For this review, take the finished solid that the model builds, in its own axes (mm). A direction names the side the tool comes from. Give positions to 0.01 mm unless a question says otherwise; leave off trailing zeros. Loops run counter-clockwise (first coordinate to the right, second up) from the corner with the lowest first, then second, coordinate; pieces in that order, holes last. Notation, with made-up numbers: (30.5, 54) - (58.5, 54) arc R28 cw to (58.5, 91) - close; hole circle Ø3 at (-21.5, 73.5). An arc over 180 degrees is marked (long way). Put each result on its own line as item: value.
from build123d import *

# Parameters (mm, degrees)
F0_W     = 935.182943
F0_H     = 745.169759
F1_DEPTH = 25
F2_W     = 160
F2_H     = 100
F3_DEPTH = 131.70007
F5_D     = 20
F6_R     = 71.842191


with BuildPart() as f1:
    # F0 (on Top) → F1 (new body)
    with BuildSketch(Plane.XY):
        with Locations((-262.850217, -86.583943)):
            Rectangle(F0_W, F0_H)
    extrude(amount=F1_DEPTH)

    # F2 (on face) → F3 (join)
    with BuildSketch(Plane.XY.offset(25)):
        with Locations((-80, -245.168384)):
            Rectangle(F2_W, F2_H)
    extrude(amount=F3_DEPTH)

    # F5 (through all)
    with Locations(Plane.XZ.offset(295.168384)):
        with Locations((-80.000006, 119.801037)):
            Hole(F5_D / 2)

    # F6
    f6_edges = [f1.edges().sort_by_distance(p)[0] for p in [
        (0, -245.168384, 156.70007),
        (-160, -245.168384, 156.70007),
    ]]
    fillet(f6_edges, radius=F6_R)


solid = f1.part
1) For faces 1 (the face through (0, -246, 55)), 2 (the face through (-81, -295.168, 90)), 3 (the face through (-730.442, -92, 12)), 4 (the face through (-160, -246, 55)), list the 3-axis set-ups (+Z, -Z, +X, -X, +Y, -Y) from which the entire face can be reached by the end or side of a thin tool; tool diameter is ignored.
Geometry check:
face 1: +Z, +X, +Y, -Y
face 2: +Z, +X, -X, -Y
face 3: +Z, -Z, -X, +Y, -Y
face 4: +Z, -X, +Y, -Y
2) Take a section at B-B on y = -247.5. State the section outline as (x, z) points.
Geometry check:
outline: (-730.44, 0) - (204.74, 0) - (204.74, 25) - (0, 25) - (0, 84.86) arc R71.84 ccw to (-71.84, 156.7) - (-88.16, 156.7) arc R71.84 ccw to (-160, 84.86) - (-160, 25) - (-730.44, 25) - close; hole circle Ø20 at (-80, 119.8)
3) Take a section at C-C on y = -145.5. State the section outline as (x, z) points.
Geometry check:
outline: (-730.44, 0) - (204.74, 0) - (204.74, 25) - (-730.44, 25) - close
4) Insertion check: pin 1 Ø6 at (x, z) = (-100, 35.5) entering from +Y; pin 2 Ø4 at (y, z) = (-195, 97) entering from +X; pin 3 Ø6 at (x, y) = (-236, 160.5) entering from -Z; pin 4 Ø4 at (x, y) = (-92.5, 122) entering from +Z. Each pin has a flat end and moves straight along its axis. Give the tip position at first contact, or say it passes through.
Geometry check:
pin 1: stops at y = -195.17
pin 2: stops at x = -0.72
pin 3: stops at z = 0
pin 4: stops at z = 25
5) Take a section at D-D on x = -351. State the section outline as (y, z) points, and give its area (3 significant figures).
Geometry check:
outline: (-459.17, 0) - (286, 0) - (286, 25) - (-459.17, 25) - close
area: 18,600 mm²
6) Draft analysis for pull direction Z (two halves, no side actions). For faces 5 (the face through (-81, -195.168, 90)), 6 (the face through (-269, -81, 0)), 7 (the face through (-20.49, -244.47, 135.1)), 8 (the face through (-84.614, -244.468, 110.929)), state which applies: pulls with the +Z half, pulls with the -Z half, needs draft (parallel to the pull), parting line crosses it, or undercut.
Geometry check:
face 5: needs draft
face 6: pulls with the -Z half
face 7: pulls with the +Z half
face 8: undercut
7) Take a section at A-A on x = -54. State the section outline as (y, z) points, and give its area (3 significant figures).
Geometry check:
outline: (-459.17, 0) - (286, 0) - (286, 25) - (-195.17, 25) - (-195.17, 154.45) - (-295.17, 154.45) - (-295.17, 25) - (-459.17, 25) - close
area: 31,600 mm²
8) Wall thickness on line 1 (Z direction, x = -213, y = 197); line 2 (Y direction, x = -54, z = 139); line 3 (X direction, y = -262, z = 99): over which ranges is each line inside the solid? List them lowest first.
Geometry check:
line 1: z = 0 to 25
line 2: y = -295.17 to -195.17
line 3: x = -158.59 to -1.41
